from build123d import *

# Parameters (mm, degrees)
F3_W           = 43
F3_H           = 43
F4_W           = 43
F4_H           = 35.5
F6_W           = 75
F6_H           = 56
F7_DEPTH       = 18
F8_R           = 5
F9_R           = 3.75
F10_DEPTH      = 8.6
F10_DEPTH_BACK = 18
F11_R          = 12
F12_DEPTH      = 16
F13_W          = 18.5
F13_H          = 16.5
F14_DEPTH      = 6


with BuildPart() as f5:
    # F3 (on offset) → F5 section 0
    with BuildSketch(Plane.XY.offset(-8.6)):
        Rectangle(F3_W, F3_H)
    # F4 (on Top) → F5 section 1
    with BuildSketch(Plane.XY):
        Rectangle(F4_W, F4_H)
    loft()

    # F6 (on Top) → F7 (join)
    with BuildSketch(Plane.XY):
        Rectangle(F6_W, F6_H)
    extrude(amount=F7_DEPTH)

    # F8
    f8_edges = [f5.edges().sort_by_distance(p)[0] for p in [
        (-37.5, 28, 9),
        (37.5, 28, 9),
        (37.5, -28, 9),
        (-37.5, -28, 9),
    ]]
    fillet(f8_edges, radius=F8_R)

    # F9 (on Top) → F10 (cut, two sides)
    with BuildSketch(Plane.XY) as f10_sk:
        with Locations((0, -4.65)):
            Circle(F9_R)
    extrude(amount=-F10_DEPTH, mode=Mode.SUBTRACT)
    extrude(f10_sk.sketch, amount=F10_DEPTH_BACK, mode=Mode.SUBTRACT)

    # F11 (on offset) → F12 (cut)
    with BuildSketch(Plane.XY.offset(-8.6)):
        with Locations((0, -4.65)):
            Circle(F11_R)
    extrude(amount=F12_DEPTH, mode=Mode.SUBTRACT)

    # F13 (on face) → F14 (cut)
    with BuildSketch(Plane.XY.offset(18)):
        with Locations((0, -4.65)):
            Rectangle(F13_W, F13_H)
    extrude(amount=-F14_DEPTH, mode=Mode.SUBTRACT)


solid = f5.part
Geometry check sheet. Reference: the model listing, model coordinates, mm. A direction names the side the tool comes from. Give positions to 0.01 mm unless a question says otherwise; leave off trailing zeros. Write each loop counter-clockwise with the first axis right and the second up, starting at its lowest first coordinate (ties: lowest second). Pieces come first, ordered by that corner, then holes. Notation, with made-up numbers: (-11.75, -25.5) - (43.25, -25.5) arc R18 cw to (43.25, 2.5) - close; hole circle Ø7 at (29.25, 59). An arc over 180 degrees is marked (long way). Put each result on its own line as item: value.
1. Sectioned sample at D-D, the plane z = 13. Enter the section's corners in (x, y).
Ans:
outline: (-37.5, -23) arc R5 ccw to (-32.5, -28) - (32.5, -28) arc R5 ccw to (37.5, -23) - (37.5, 23) arc R5 ccw to (32.5, 28) - (-32.5, 28) arc R5 ccw to (-37.5, 23) - close; hole (-9.25, -12.9) - (9.25, -12.9) - (9.25, 3.6) - (-9.25, 3.6) - close
2. Go/stop test with flat-tipped pins: pin 1 (8 mm diameter, centred on y = 5, z = -4.5, fed in from -X); pin 2 (14.5 mm diameter, centred on x = 0, y = -4.65, fed in from +Z); pin 3 (4.5 mm diameter, centred on x = 0, y = -4.65, fed in from -Z); pin 4 (1.5 mm diameter, centred on x = -11.5, z = -2, fed in from +Y). Record where each tip stops, or that it passes through.
Ans:
pin 1: stops at x = -21.5
pin 2: stops at z = 12
pin 3: passes through
pin 4: stops at y = 18.95
3. Sectioned sample at C-C, the plane x = -19. Enter the section's corners in (y, z), plus the area to 3 significant figures.
Ans:
outline: (-28, 0) - (-17.75, 0) - (-21.5, -8.6) - (21.5, -8.6) - (17.75, 0) - (28, 0) - (28, 18) - (-28, 18) - close
area: 1,350 mm²
4. Sectioned sample at B-B, the plane z = 1. Enter the section's corners in (x, y), plus the area to 3 significant figures.
Ans:
outline: (-37.5, -23) arc R5 ccw to (-32.5, -28) - (32.5, -28) arc R5 ccw to (37.5, -23) - (37.5, 23) arc R5 ccw to (32.5, 28) - (-32.5, 28) arc R5 ccw to (-37.5, 23) - close; hole circle Ø24 at (0, -4.65)
area: 3,730 mm²
5. Thickness scan on line 1 (Y direction, x = 0, z = 0.5); line 2 (Y direction, x = 0, z = 9.35); line 3 (X direction, y = -4.65, z = 9.25). Record the ranges inside material, lowest first.
Ans:
line 1: y = -28 to -16.65, 7.35 to 28
line 2: y = -28 to -8.4, -0.9 to 28
line 3: x = -37.5 to -3.75, 3.75 to 37.5
6. Draft check along Z on faces 1 (the flat face through (-9.25, -5, 15)), 2 (the flat face through (-3, -2, 7.4)), 3 (the flat face through (0.3, 19.6, -4.24)). Enter one of: +Z half, -Z half, draft (parallel to the pull), parting line (faces both ways), or undercut.
Ans:
face 1: draft
face 2: -Z half
face 3: undercut
7. Set-up check for faces 4 (the flat face through (-1, 19, 0)), 5 (the flat face through (9.25, -5, 15)), 6 (the cylindrical face through (-11.99, -4.12, -0.71)): record each of +Z, -Z, +X, -X, +Y, -Y from which the full face is reachable in a straight line by a thin tool's end or side.
Ans:
face 4: none
face 5: +Z
face 6: -Z
8. Sectioned sample at A-A, the plane x = 0. Enter the section's corners in (y, z), plus the area to 3 significant figures.
Ans:
outline: (-28, 0) - (-17.75, 0) - (-21.5, -8.6) - (-16.65, -8.6) - (-16.65, 7.4) - (-8.4, 7.4) - (-8.4, 12) - (-12.9, 12) - (-12.9, 18) - (-28, 18) - close; (-0.9, 7.4) - (7.35, 7.4) - (7.35, -8.6) - (21.5, -8.6) - (17.75, 0) - (28, 0) - (28, 18) - (3.6, 18) - (3.6, 12) - (-0.9, 12) - close
area: 828 mm²
